from build123d import *

# Parameters (mm, degrees)
CYLINDER2353_R         = 17
CYLINDER2353_DEPTH     = 160
CYLINDER2410_R         = 60.2
CYLINDER2410_DEPTH     = 58
BOX593_W               = 6
BOX593_H               = 6
BOX593_DEPTH           = 64
BOX592_W               = 6
BOX592_H               = 6
BOX592_DEPTH           = 64
CYLINDER2386_R         = 3
CYLINDER2386_DEPTH     = 3
CYLINDER2368_R         = 3
CYLINDER2368_DEPTH     = 3
CYLINDER2394_R         = 1.5
CYLINDER2394_DEPTH     = 32
CYLINDER2392_R         = 1.5
CYLINDER2392_DEPTH     = 32
CYLINDER2391_R         = 1.5
CYLINDER2391_DEPTH     = 100
CYLINDER2406_R         = 1.5
CYLINDER2406_DEPTH     = 100
CYLINDER2396_R         = 1.5
CYLINDER2396_DEPTH     = 50
CYLINDER2393_R         = 1.5
CYLINDER2393_DEPTH     = 50
CYLINDER2389_R         = 1.5
CYLINDER2389_DEPTH     = 50
CYLINDER2398_R         = 1.5
CYLINDER2398_DEPTH     = 50
CYLINDER2379_R         = 1.5
CYLINDER2379_DEPTH     = 100
CYLINDER2399_R         = 1.5
CYLINDER2399_DEPTH     = 100
CYLINDER2401_R         = 1.5
CYLINDER2401_DEPTH     = 100
CYLINDER2405_R         = 1.5
CYLINDER2405_DEPTH     = 100
BOX590_W               = 200
BOX590_H               = 100
BOX590_DEPTH           = 32
TUBE096_R              = 59
TUBE096_R_2            = 40
TUBE096_DEPTH          = 10
CUT574_PLACEMENT_ANGLE = 180
FILLET047_R            = 8


with BuildPart() as obj1:
    # Cylinder2353 → Cylinder2353 (new body)
    with BuildSketch(Plane(origin=(-18, 0, -60), x_dir=(1, 0, 0), z_dir=(0, 0, 1))):
        Circle(CYLINDER2353_R)
    extrude(amount=CYLINDER2353_DEPTH)


with BuildPart() as obj2:
    # Cylinder2410 → Cylinder2410 (new body)
    with BuildSketch(Plane(origin=(0, 19, -53), x_dir=(1, 0, 0), z_dir=(0, -1, 0))):
        Circle(CYLINDER2410_R)
    extrude(amount=CYLINDER2410_DEPTH)


with BuildPart() as krychle593:
    # Box593 → Box593 (new body)
    with BuildSketch(Plane(origin=(87, -3, -93), x_dir=(1, 0, 0), z_dir=(0, 0, 1))):
        with Locations((3, 3)):
            Rectangle(BOX593_W, BOX593_H)
    extrude(amount=BOX593_DEPTH)


with BuildPart() as compound1005:
    # Box592 → Box592 (new body)
    with BuildSketch(Plane(origin=(11, -3, -93), x_dir=(1, 0, 0), z_dir=(0, 0, 1))):
        with Locations((3, 3)):
            Rectangle(BOX592_W, BOX592_H)
    extrude(amount=BOX592_DEPTH)

    # Compound1005: union Krychle593
    add(krychle593.part)


with BuildPart() as compound1005_1:
    # Compound1005 placement: moved
    add(compound1005.part.moved(Location((-52, 0, 36))))


with BuildPart() as obj3:
    # Cylinder2386 → Cylinder2386 (new body)
    with BuildSketch(Plane(origin=(78, 41, -42), x_dir=(1, 0, 0), z_dir=(0, 0, 1))):
        Circle(CYLINDER2386_R)
    extrude(amount=CYLINDER2386_DEPTH)


with BuildPart() as compound1002:
    # Cylinder2368 → Cylinder2368 (new body)
    with BuildSketch(Plane(origin=(26, 41, -42), x_dir=(1, 0, 0), z_dir=(0, 0, 1))):
        Circle(CYLINDER2368_R)
    extrude(amount=CYLINDER2368_DEPTH)

    # Compound1002: union obj3
    add(obj3.part)


with BuildPart() as compound1002_1:
    # Compound1002 placement: moved
    add(compound1002.part.moved(Location((-52, 0, 42))))


with BuildPart() as obj4:
    # Cylinder2394 → Cylinder2394 (new body)
    with BuildSketch(Plane(origin=(78, 41, -42), x_dir=(1, 0, 0), z_dir=(0, 0, 1))):
        Circle(CYLINDER2394_R)
    extrude(amount=CYLINDER2394_DEPTH)


with BuildPart() as compound1008:
    # Cylinder2392 → Cylinder2392 (new body)
    with BuildSketch(Plane(origin=(26, 41, -42), x_dir=(1, 0, 0), z_dir=(0, 0, 1))):
        Circle(CYLINDER2392_R)
    extrude(amount=CYLINDER2392_DEPTH)

    # Compound1008: union obj4
    add(obj4.part)


with BuildPart() as compound1008_1:
    # Compound1008 placement: moved
    add(compound1008.part.moved(Location((-52, 0, 36))))


with BuildPart() as obj5:
    # Cylinder2391 → Cylinder2391 (new body)
    with BuildSketch(Plane(origin=(14, 0, -60), x_dir=(1, 0, 0), z_dir=(0, 0, 1))):
        Circle(CYLINDER2391_R)
    extrude(amount=CYLINDER2391_DEPTH)


with BuildPart() as compound1006:
    # Cylinder2406 → Cylinder2406 (new body)
    with BuildSketch(Plane(origin=(90, 0, -60), x_dir=(1, 0, 0), z_dir=(0, 0, 1))):
        Circle(CYLINDER2406_R)
    extrude(amount=CYLINDER2406_DEPTH)

    # Compound1022: union obj5
    add(obj5.part)


with BuildPart() as compound1006_1:
    # Compound1022 placement: moved
    add(compound1006.part.moved(Location((-52, 0, 0))))

    # Compound1006: union Compound1008
    add(compound1008_1.part)


with BuildPart() as obj6:
    # Cylinder2396 → Cylinder2396 (new body)
    with BuildSketch(Plane(origin=(-51, 6, 0), x_dir=(1, 0, 0), z_dir=(0, 0, 1))):
        Circle(CYLINDER2396_R)
    extrude(amount=CYLINDER2396_DEPTH)


with BuildPart() as obj7:
    # Cylinder2393 → Cylinder2393 (new body)
    with BuildSketch(Plane(origin=(-24, 18, 0), x_dir=(1, 0, 0), z_dir=(0, 0, 1))):
        Circle(CYLINDER2393_R)
    extrude(amount=CYLINDER2393_DEPTH)


with BuildPart() as obj8:
    # Cylinder2389 → Cylinder2389 (new body)
    with BuildSketch(Plane(origin=(24, 18, 0), x_dir=(1, 0, 0), z_dir=(0, 0, 1))):
        Circle(CYLINDER2389_R)
    extrude(amount=CYLINDER2389_DEPTH)


with BuildPart() as compound1015:
    # Cylinder2398 → Cylinder2398 (new body)
    with BuildSketch(Plane(origin=(51, 6, 0), x_dir=(1, 0, 0), z_dir=(0, 0, 1))):
        Circle(CYLINDER2398_R)
    extrude(amount=CYLINDER2398_DEPTH)

    # Compound1015: union obj6, obj7, obj8
    add(obj6.part)
    add(obj7.part)
    add(obj8.part)


with BuildPart() as compound1015_1:
    # Compound1015 placement: moved
    add(compound1015.part.moved(Location((0, 6, 0))))


with BuildPart() as obj9:
    # Cylinder2379 → Cylinder2379 (new body)
    with BuildSketch(Plane(origin=(51, -12, 0), x_dir=(1, 0, 0), z_dir=(0, 0, 1))):
        Circle(CYLINDER2379_R)
    extrude(amount=CYLINDER2379_DEPTH)


with BuildPart() as compound997:
    # Cylinder2399 → Cylinder2399 (new body)
    with BuildSketch(Plane(origin=(-51, -12, 0), x_dir=(1, 0, 0), z_dir=(0, 0, 1))):
        Circle(CYLINDER2399_R)
    extrude(amount=CYLINDER2399_DEPTH)

    # Compound997: union obj9
    add(obj9.part)


with BuildPart() as obj10:
    # Cylinder2401 → Cylinder2401 (new body)
    with BuildSketch(Plane(origin=(39, -21, 0), x_dir=(1, 0, 0), z_dir=(0, 0, 1))):
        Circle(CYLINDER2401_R)
    extrude(amount=CYLINDER2401_DEPTH)


with BuildPart() as compound1018:
    # Cylinder2405 → Cylinder2405 (new body)
    with BuildSketch(Plane(origin=(-39, -21, 0), x_dir=(1, 0, 0), z_dir=(0, 0, 1))):
        Circle(CYLINDER2405_R)
    extrude(amount=CYLINDER2405_DEPTH)

    # Compound1017: union obj10
    add(obj10.part)


with BuildPart() as compound1018_1:
    # Compound1017 placement: moved
    add(compound1018.part.moved(Location((0, -6, 0))))

    # Compound1018: union Compound1015, Compound997
    add(compound1015_1.part)
    add(compound997.part)


with BuildPart() as compound1018_2:
    # Compound1018 placement: moved
    add(compound1018_1.part.moved(Location((0, 0, -10))))


with BuildPart() as krychle590:
    # Box590 → Box590 (new body)
    with BuildSketch(Plane(origin=(-100, -130, 0), x_dir=(1, 0, 0), z_dir=(0, 0, 1))):
        with Locations((100, 50)):
            Rectangle(BOX590_W, BOX590_H)
    extrude(amount=BOX590_DEPTH)


with BuildPart() as fillet047:
    # Tube096 → Tube096 (new body)
    with BuildSketch(Plane.XY):
        Circle(TUBE096_R)
        Circle(TUBE096_R_2, mode=Mode.SUBTRACT)
    extrude(amount=TUBE096_DEPTH)

    # Cut575: cut Krychle590
    add(krychle590.part, mode=Mode.SUBTRACT)

    # Cut591: cut Compound1018
    add(compound1018_2.part, mode=Mode.SUBTRACT)

    # Cut585: cut Compound1006
    add(compound1006_1.part, mode=Mode.SUBTRACT)

    # Cut578: cut Compound1002
    add(compound1002_1.part, mode=Mode.SUBTRACT)

    # Cut592: cut Compound1005
    add(compound1005_1.part, mode=Mode.SUBTRACT)

    # Cut574: cut obj2
    add(obj2.part, mode=Mode.SUBTRACT)


with BuildPart() as fillet047_1:
    # Cut574 placement: moved
    add(fillet047.part.moved(Location((52, 0, -36))).rotate(Axis((52, 0, -36), (0, 0, 1)), CUT574_PLACEMENT_ANGLE))

    # Cut593: cut obj1
    add(obj1.part, mode=Mode.SUBTRACT)

    # Fillet047
    fillet047_edges = [fillet047_1.edges().sort_by_distance(p)[0] for p in [
        (-5.8, 11.838919, -31),
        (-5.8, -11.838919, -31),
    ]]
    fillet(fillet047_edges, radius=FILLET047_R)


solid = fillet047_1.part
CAD build for the part. Positions are in the model's coordinates, mm. A direction names the side the tool comes from. Coordinates: 2 decimals unless noted, no trailing zeros. Order: outer loops, then holes, each group sorted by start corner. A loop starts at its lowest first (then second) coordinate and runs counter-clockwise, first axis right, second up.
Item 1: Pin check, flat tips, straight feed: pin 1 Ø1.8 at (x, y) = (91, 27) entering from +Z; pin 2 Ø1.8 at (x, y) = (77, -42) entering from -Z; pin 3 Ø0.9 at (x, z) = (92.5, -33.5) entering from -Y; pin 4 Ø4 at (y, z) = (-1, -35) entering from -X. Stop position of each tip, or through.
Check sheet entries:
pin 1: passes through
pin 2: stops at z = -33
pin 3: stops at y = -43.32
pin 4: stops at x = -1.27
Item 2: Two-plate mould, pull along Y, no slides. Class faces 1 (the face through (54, -45, -36)), 2 (the face through (-2.23, 23.24, -31.07)), 3 (the face through (76.7, -39.7, -33)): +Y half, -Y half, draft (parallel to the pull), parting line (faces both ways), or undercut.
Check sheet entries:
face 1: draft
face 2: +Y half
face 3: undercut
Item 3: Band-saw the part on D-D on x = 69.5. List the corners of the cut face in (y, z).
Check sheet entries:
outline: (-56.34, -36) - (-35.97, -36) - (-35.97, -26) - (-56.34, -26) - close
Item 4: 3-axis set-ups, long thin cutter, end or side, ignore diameter. For faces 4 (the face through (93, 0, -33)), 5 (the face through (-1, 0, -31)): which of +Z, -Z, +X, -X, +Y, -Y reach the whole face in a straight line?
Check sheet entries:
face 4: -Z
face 5: +Z, -Z, -X
Item 5: Band-saw the part on B-B on x = 87.5. List the corners of the cut face in (y, z).
Check sheet entries:
outline: (-47.12, -36) - (-18.43, -36) - (-18.43, -26) - (-47.12, -26) - close; (18.43, -36) - (30, -36) - (30, -26) - (18.43, -26) - close
Item 6: Band-saw the part on C-C on z = -27.5. Give the number of separate pieces and of enclosed holes in the cut face, plus the area to 3 significant figures.
Check sheet entries:
separate pieces: 1
enclosed holes: 8
area: 4,030 mm2
Item 7: Drill centre lines: L1, parallel to X at y = -41, z = -34.55; L2, parallel to Y at x = 24, z = -33.75; L3, parallel to Y at x = 1, z = -32. Where is each one in solid material? Low to high.
Check sheet entries:
L1: x = 9.57 to 23, 29 to 75, 81 to 94.43
L2: y = -51.93 to -43.24, -38.76 to -28.57, 28.57 to 30
L3: y = -29.66 to -13.5, -10.5 to 10.5, 13.5 to 29.66
Item 8: Band-saw the part on A-A on y = 6. List the corners of the cut face in (x, z).
Check sheet entries:
outline: (-2.09, -36) - (12.45, -36) - (12.45, -26) - (-2.09, -26) - close; (91.55, -36) - (110.69, -36) - (110.69, -26) - (91.55, -26) - close
